from build123d import *

# Parameters (mm, degrees)
SKETCH1_W                   = 120.4
SKETCH1_H                   = 10
DODANIE_WYCI_GNI_CIE1_DEPTH = 125
SZKIC1_R                    = 2
WYTNIJ_WYCI_GNI_CIE1_DEPTH  = 10
WYTNIJ_WYCI_GNI_CIE2_START  = -10
SZKIC2_R                    = 2
WYTNIJ_WYCI_GNI_CIE2_DEPTH  = 10
SZKIC3_R                    = 2
WYTNIJ_WYCI_GNI_CIE3_DEPTH  = 10
WYTNIJ_WYCI_GNI_CIE4_START  = -10
SZKIC4_R                    = 2
WYTNIJ_WYCI_GNI_CIE4_DEPTH  = 10


with BuildPart() as part:
    # Sketch1 → Dodanie-wyciągnięcie1 (new body)
    with BuildSketch(Plane(origin=(0, 0, 0), x_dir=(1, 0, 0), z_dir=(0, 1, 0))):
        with Locations((60.2, 5)):
            Rectangle(SKETCH1_W, SKETCH1_H)
    extrude(amount=DODANIE_WYCI_GNI_CIE1_DEPTH)

    # Szkic1 → Wytnij-wyciągnięcie1 (cut)
    with BuildSketch(Plane(origin=(0, 125, 0), x_dir=(1, 0, 0), z_dir=(0, 1, 0))):
        with Locations(Location((15.2, 5, 0), (0, 0, 270))):
            Circle(SZKIC1_R)
        with Locations(Location((60.2, 5, 0), (0, 0, 270))):
            Circle(SZKIC1_R)
        with Locations(Location((105.2, 5, 0), (0, 0, 270))):
            Circle(SZKIC1_R)
    extrude(amount=-WYTNIJ_WYCI_GNI_CIE1_DEPTH, mode=Mode.SUBTRACT)

    # Szkic2 → Wytnij-wyciągnięcie2 (cut)
    with BuildSketch(Plane.XZ.offset(WYTNIJ_WYCI_GNI_CIE2_START)):
        with Locations(Location((15.2, -5, 0), (0, 0, 90))):
            Circle(SZKIC2_R)
        with Locations(Location((60.2, -5, 0), (0, 0, 90))):
            Circle(SZKIC2_R)
        with Locations(Location((105.2, -5, 0), (0, 0, 90))):
            Circle(SZKIC2_R)
    extrude(amount=WYTNIJ_WYCI_GNI_CIE2_DEPTH, mode=Mode.SUBTRACT)

    # Szkic3 → Wytnij-wyciągnięcie3 (cut)
    with BuildSketch(Plane.ZY):
        with Locations((-5, 93.75)):
            Circle(SZKIC3_R)
        with Locations((-5, 31.25)):
            Circle(SZKIC3_R)
    extrude(amount=-WYTNIJ_WYCI_GNI_CIE3_DEPTH, mode=Mode.SUBTRACT)

    # Szkic4 → Wytnij-wyciągnięcie4 (cut)
    with BuildSketch(Plane(origin=(120.4, 0, 0), x_dir=(0, 0, -1), z_dir=(1, 0, 0)).offset(WYTNIJ_WYCI_GNI_CIE4_START)):
        with Locations(Location((5, 93.75, 0), (0, 0, 180))):
            Circle(SZKIC4_R)
        with Locations(Location((5, 31.25, 0), (0, 0, 180))):
            Circle(SZKIC4_R)
    extrude(amount=WYTNIJ_WYCI_GNI_CIE4_DEPTH, mode=Mode.SUBTRACT)


solid = part.part
The model under review builds one solid part; all positions refer to its coordinate system, in mm. A direction names the side the tool comes from. Round coordinates to 2 decimals unless told otherwise and drop trailing zeros. Write each loop counter-clockwise with the first axis right and the second up, starting at its lowest first coordinate (ties: lowest second). Pieces come first, ordered by that corner, then holes. Notation, with made-up numbers: M 66.5,12.25 L 100.5,12.25 A20 cw 100.5,42.25 Z; hole C 29,63 d11. An arc over 180 degrees is marked long. Use a Markdown table: item, result. Add a question column.
Q1. Insertion check: pin 1 (3 mm diameter, centred on x = 105, z = -5, fed in from -Y); pin 2 (1.2 mm diameter, centred on y = 93.5, z = -5, fed in from +X); pin 3 (2 mm diameter, centred on x = 61, z = -5.5, fed in from +Y). Each pin has a flat end and moves straight along its axis. Give the tip position at first contact, or say it passes through.
Q2. To check wall thickness, follow line 1 (X direction, y = 118.5, z = -5); line 2 (Y direction, x = 7.25, z = -5); line 3 (Z direction, x = 116.25, y = 93.75). State the ranges of each line that lie inside material, in increasing order.
Q3. Machinability: for faces 1 (the face through (58.426, 120.07, -4.077)), 2 (the face through (115.33, 33.202, -5.434)), 3 (the face through (4.93, 29.298, -5.434)), which of the approach directions +Z, -Z, +X, -X, +Y, -Y give a long, thin tool a straight path to every point of the face, cutting with its end or side? Answer none if there is none.
Q4. The part is to be moulded in two halves that separate along Z. For faces 4 (the face through (120.4, 62, -5)), 5 (the face through (15, 115, -5)), 6 (the face through (59, 62, 0)), 7 (the face through (58.217, 5.07, -5.26)), say which applies: pulls with the +Z half, pulls with the -Z half, needs draft (parallel to the pull), parting line crosses it, or undercut.
Q5. We need section A-A, the plane x = 105.2. State the section outline as (y, z) points.
Findings below:
| question | item | result |
|---|---|---|
| 1 | pin 1 | stops at y = 10 |
| 1 | pin 2 | stops at x = 110.4 |
| 1 | pin 3 | stops at y = 115 |
| 2 | line 1 | x = 0 to 13.2, 17.2 to 58.2, 62.2 to 103.2, 107.2 to 120.4 |
| 2 | line 2 | y = 0 to 29.25, 33.25 to 91.75, 95.75 to 125 |
| 2 | line 3 | z = -10 to -7, -3 to 0 |
| 3 | face 1 | +Y |
| 3 | face 2 | +X |
| 3 | face 3 | -X |
| 4 | face 4 | needs draft |
| 4 | face 5 | undercut |
| 4 | face 6 | pulls with the +Z half |
| 4 | face 7 | undercut |
| 5 | outline | M 0,-10 L 125,-10 L 125,-7 L 115,-7 L 115,-3 L 125,-3 L 125,0 L 0,0 L 0,-3 L 10,-3 L 10,-7 L 0,-7 Z |
